Autodesk Inventor part; units mm, degrees
ref_plane "YZ Plane" through (0, 0, 0) normal (1, 0, 0) x (0, 1, 0)
ref_plane "XZ Plane" through (0, 0, 0) normal (0, 1, 0) x (-1, 0, 0)
ref_plane "XY Plane" through (0, 0, 0) normal (0, 0, 1) x (1, 0, 0)
sketch "스케치1" plane through (0, 0, 0) normal (0, 1, 0) x (-1, 0, 0)
  line L0 (21.7693, 2.842) -> (-28.2307, 2.842)
  line L1 (-28.2307, 2.842) -> (-28.2307, -0.158)
  line L2 (-28.2307, -0.158) -> (21.7693, -0.158)
  line L3 (21.7693, -0.158) -> (21.7693, 2.842)
  line L4 (21.7693, 4.842) -> (-28.2307, 4.842)
  line L5 (-28.2307, 4.842) -> (-28.2307, -4.158)
  line L6 (-28.2307, -4.158) -> (21.7693, -4.158)
  line L7 (21.7693, -4.158) -> (21.7693, 4.842)
  line L8 (-28.2307, 4.842) -> (-38.2307, 4.842)
  line L9 (-38.2307, 4.842) -> (-38.2307, -5.158)
  line L10 (-38.2307, -5.158) -> (-28.2307, -5.158)
  line L11 (-28.2307, -5.158) -> (-28.2307, 4.842)
  line L12 (21.7693, 4.842) -> (31.7693, 4.842)
  line L13 (31.7693, 4.842) -> (31.7693, -5.158)
  line L14 (31.7693, -5.158) -> (21.7693, -5.158)
  line L15 (21.7693, -5.158) -> (21.7693, 4.842)
  circle A0 centre (26.7693, -0.158) radius 1.75
  circle A1 centre (-33.2307, -0.158) radius 1.75
  line L16 (18.7693, 2.842) -> (18.7693, -4.158)
  line L17 (-25.2307, 2.842) -> (-25.2307, -4.158)
  line L18 (-28.2307, 0.842) -> (21.7693, 0.842)
  line L19 (21.7693, 0.842) -> (21.7693, -2.158)
  line L20 (21.7693, -2.158) -> (-28.2307, -2.158)
  line L21 (-28.2307, -2.158) -> (-28.2307, 0.842)
  point P0 (0, 0)
  point P1 (-28.2307, 2.842)
  point P2 (-25.2307, 0.842)
  point P3 (-25.2307, -2.158)
  point P4 (18.7693, -2.158)
  point P5 (18.7693, 0.842)
  dimension "d0" = 50
  dimension "d1" = 3
  dimension "d2" = 10
  dimension "d3" = 10
  dimension "d4" = 0
  dimension "d5" = 2
  dimension "d6" = 10
  dimension "d7" = 10
  dimension "d8" = 0
  dimension "d9" = 3.5
  dimension "d10" = 3.5
  dimension "d11" = 5
  dimension "d12" = 5
  dimension "d13" = 5
  dimension "d14" = 5
  dimension "d15" = 3
  dimension "d16" = 2
  dimension "d17" = 2
  dimension "d18" = 3
  dimension "d19" = 3
extrude "돌출1" add sketch "스케치1" along normal blind 10 contours L7 L12 L13 L14 L15 L3 | L5 L1 L11 L10 L9 L8 | A0 | A1
extrude "돌출2" add sketch "스케치1" along normal blind 10 contours L3 L18 L16 L0 | L17 L18 L1 L0 | L7 L6 L16 L20 | L17 L6 L5 L20
extrude "돌출3" add sketch "스케치1" along normal blind 3 contours L3 L2 L16 L18 | L16 L2 L17 L18 | L7 L20 L16 L2 | L17 L2 L1 L18 | L16 L20 L17 L2 | L17 L20 L5 L2
extrude "돌출4" add sketch "스케치1" along normal blind 6 contours L16 L18 L17 L0 | L16 L6 L17 L20
fillet "모깎기1" radius 2 4 edges at (28.2307, 5, -4.158) (-21.7693, 5, -4.158) (28.2307, 5, 2.842) (-21.7693, 5, 2.842)
sketch "스케치4" plane through (28.2307, 10, -2.158) normal (-1, 0, 0) x (0, 0, 1)
  point P0 (2.158, -10)
equation "\"d3\" = d2"
equation "\"d7\" = d6"
equation "\"d12\" = d11"
equation "\"d14\" = d13"
properties part number "B5-camera-fu"
Design review of the part built by this model. Coordinates are the model's own, in mm. A direction names the side the tool comes from. Give positions to 0.01 mm unless a question says otherwise; leave off trailing zeros. Order: outer loops, then holes, each group sorted by start corner. A loop starts at its lowest first (then second) coordinate and runs counter-clockwise, first axis right, second up.
1. Add section A-A, the plane y = 7.25. State the section outline as (x, z) points, then the cut area to 3 significant figures.
Solution:
outline: (-31.77, -5.16) - (-21.77, -5.16) arc R2 cw to (-20.04, -4.16) - (-18.77, -4.16) - (-18.77, -2.16) - (-21.77, -2.16) - (-21.77, 0.84) - (-18.77, 0.84) - (-18.77, 2.84) - (-19.77, 2.84) arc R2 cw to (-21.77, 4.84) - (-31.77, 4.84) - close; (25.23, -4.16) - (26.5, -4.16) arc R2 cw to (28.23, -5.16) - (38.23, -5.16) - (38.23, 4.84) - (28.23, 4.84) arc R2 cw to (26.23, 2.84) - (25.23, 2.84) - (25.23, 0.84) - (28.23, 0.84) - (28.23, -2.16) - (25.23, -2.16) - close
area: 227 mm2
2. To check wall thickness, follow L1, parallel to X at y = 9.5, z = 1.5; L2, parallel to X at y = 9.5, z = -0.25; L3, parallel to Z at x = -10, y = 3.75. State the ranges of each line that lie inside material, in increasing order.
Solution:
L1: x = -31.77 to -18.77, 25.23 to 38.23
L2: x = -31.77 to -21.77, 28.23 to 38.23
L3: z = -4.16 to -2.16, 0.84 to 2.84
3. Add section B-B, the plane z = 3.5. State the section outline as (x, y) points.
Solution:
outline: (-31.77, 0) - (-21.25, 0) - (-21.25, 10) - (-31.77, 10) - close; (27.71, 0) - (38.23, 0) - (38.23, 10) - (27.71, 10) - close
4. Mouldability with a two-part tool opening along X and no side actions: class faces 5 (the flat face through (38.231, 5, 0)), 6 (the flat face through (-31.769, 5, 0)), 7 (the flat face through (25.231, 8, 2)) as +X half, -X half, draft (parallel to the pull), parting line (faces both ways), or undercut.
Solution:
face 5: +X half
face 6: -X half
face 7: undercut
5. Tool access review of faces 1 (the flat face through (3, 5, -2.158)), 2 (the flat face through (4, 6, 2)), 3 (the flat face through (4, 3, -4.158)), 4 (the flat face through (3, 3, 2.842)): name each direction out of +Z, -Z, +X, -X, +Y, -Y from which nothing blocks a thin tool from reaching the whole face with its end or side.
Solution:
face 1: +Y
face 2: +Z, -Z, +Y
face 3: -Z, +Y, -Y
face 4: +Z, +Y, -Y
6. Add section C-C, the plane y = 1.25. State the section outline as (x, z) points.
Solution:
outline: (-31.77, -5.16) - (-21.77, -5.16) arc R2 cw to (-20.04, -4.16) - (26.5, -4.16) arc R2 cw to (28.23, -5.16) - (38.23, -5.16) - (38.23, 4.84) - (28.23, 4.84) arc R2 cw to (26.23, 2.84) - (-19.77, 2.84) arc R2 cw to (-21.77, 4.84) - (-31.77, 4.84) - close
7. Add section D-D, the plane x = 18. State the section outline as (y, z) points, then the cut area to 3 significant figures.
Solution:
outline: (0, -4.16) - (6, -4.16) - (6, -2.16) - (3, -2.16) - (3, 0.84) - (6, 0.84) - (6, 2.84) - (0, 2.84) - close
area: 33.0 mm2
8. For pin 1 Ø1.5 at (x, y) = (24.5, 6.5) entering from -Z; pin 2 Ø1.6 at (x, z) = (-2, -3.5) entering from +Y; pin 3 Ø4 at (x, y) = (16, 2.5) entering from +Z, all flat-tipped, find the tip position at first contact; note any pin that passes through.
Solution:
pin 1: stops at z = -4.16
pin 2: stops at y = 6
pin 3: stops at z = 2.84
